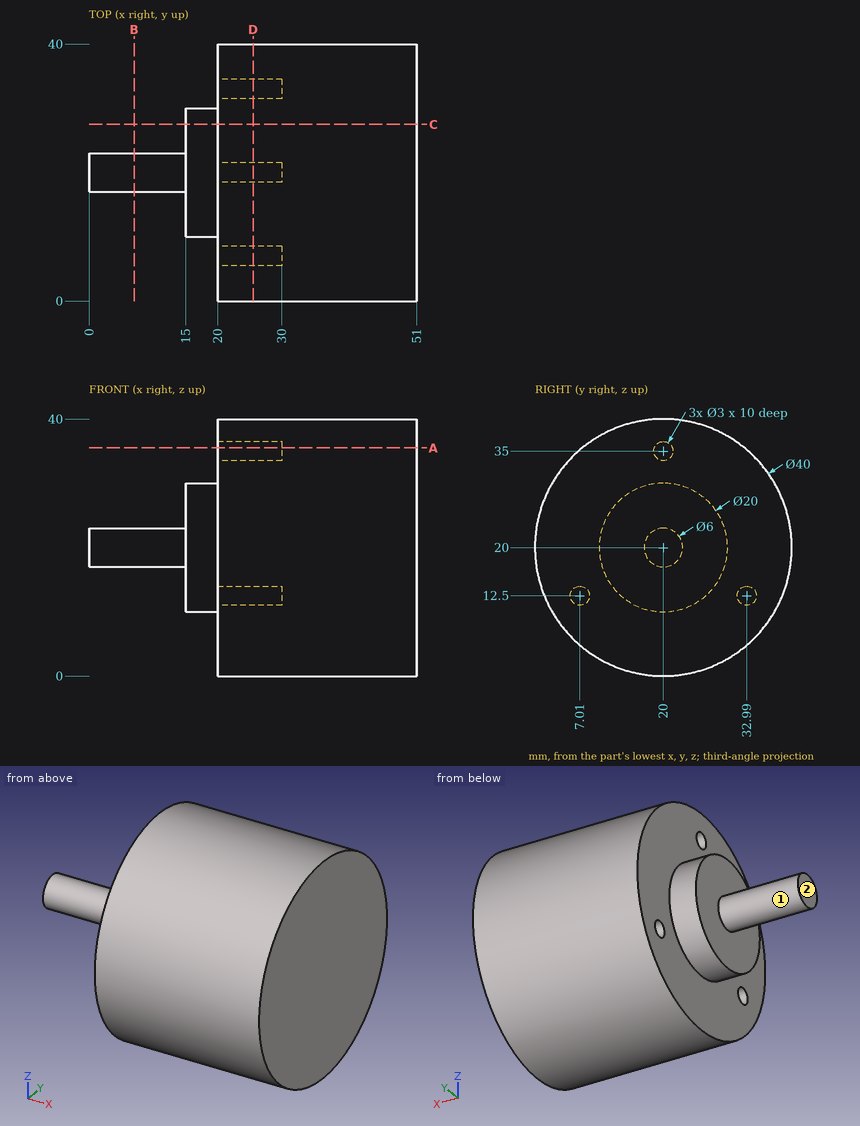
Geometry: see drawing. Coordinates: mm, zero at the bounding-box minimum. A direction names the side the tool comes from. Give positions to 0.01 mm unless a question says otherwise; leave off trailing zeros. Loops run counter-clockwise (first coordinate to the right, second up) from the corner with the lowest first, then second, coordinate; pieces in that order, holes last. Notation, with made-up numbers: (20.5, -12.5) -> (25.5, -12.5) arc R27 cw to (25.5, 21.5) -> close; hole circle Ø11 at (-28, 72.5). An arc over 180 degrees is marked (long way). Use CSV: the item, a comma, the result in double quotes.
(1) Cut plane A-A (z = 35.5). Output: boundary loops of the cut face in (x, y), plus the area to 3 significant figures.
From the geometry:
outline,"(20, 7.36) -> (51, 7.36) -> (51, 32.64) -> (20, 32.64) -> (20, 21.41) -> (30, 21.41) -> (30, 18.59) -> (20, 18.59) -> close"
area,"755 mm^2"
(2) First-contact query: P1, Ø3, axis at x = 40.5, z = 6.5, coming from the -Y side; P2, Ø3, axis at x = 16, z = 28, coming from the +Y side; P3, Ø2.5, axis at y = 32.99, z = 12.5, coming from the -X side; P4, Ø16, axis at y = 21.5, z = 22, coming from the -X side. Flat tips, straight axial feed; report the tip coordinate or a pass-through.
From the geometry:
P1,"y = 4"
P2,"y = 27.6"
P3,"x = 30"
P4,"x = 0"
(3) Cut plane C-C (y = 27.5). Output: boundary loops of the cut face in (x, z) (1 decimal), plus the area to 3 significant figures.
From the geometry:
outline,"(15, 13.4) -> (20, 13.4) -> (20, 1.5) -> (51, 1.5) -> (51, 38.5) -> (20, 38.5) -> (20, 26.6) -> (15, 26.6) -> close"
area,"1,220 mm^2"
(4) Cut plane D-D (x = 25.5). Output: boundary loops of the cut face in (y, z).
From the geometry:
outline,"circle Ø40 at (20, 20); hole circle Ø3 at (7.01, 12.5); hole circle Ø3 at (20, 35); hole circle Ø3 at (32.99, 12.5)"
(5) Cut plane B-B (x = 7). Output: boundary loops of the cut face in (y, z).
From the geometry:
outline,"circle Ø6 at (20, 20)"
(6) Access query for the marked faces 1 and 2. Directions: +Z, -Z, +X, -X, +Y, -Y. A direction counts if a zero-diameter tool reaches every point of the face in a straight line with its end or side. Return the directions, or none.
From the geometry:
face 1,"-X"
face 2,"+Z, -Z, -X, +Y, -Y"
(7) Ray query, line 1 along Y through (x, z) = (24.75, 12.5); line 2 along X through (y, z) = (12.5, 18); line 3 along X through (y, z) = (13, 29). Return the intervals inside material, ascending. Write a range as [from, to].
From the geometry:
line 1,"[1.46, 5.51], [8.51, 31.49], [34.49, 38.54]"
line 2,"[15, 51]"
line 3,"[20, 51]"
